Read the model definition and answer for the solid it produces. Units are mm, in the model's axes. A direction names the side the tool comes from. Coordinates: 2 decimals unless noted, no trailing zeros. Write each loop counter-clockwise with the first axis right and the second up, starting at its lowest first coordinate (ties: lowest second). Pieces come first, ordered by that corner, then holes. Notation, with made-up numbers: (-34.5, 71) -> (9.5, 71) arc R29 cw to (9.5, 110) -> close; hole circle Ø9 at (68, 62). An arc over 180 degrees is marked (long way). Return JSON: item names as keys, results as strings.
from build123d import *

# Parameters (mm, degrees)
F0_W     = 38.1
F0_H     = 25.4
F1_DEPTH = 12.7
F2_W     = 25.409764
F2_H     = 17.182311
F3_DEPTH = 25.401
F5_DEPTH = 38.101


with BuildPart() as f1:
    # F0 (on Front) → F1 (new body, symmetric)
    with BuildSketch(Plane.XZ):
        with Locations((19.05, 12.7)):
            Rectangle(F0_W, F0_H)
    extrude(amount=F1_DEPTH, both=True)

    # F2 (on face) → F3 (cut, through all)
    with BuildSketch(Plane.XZ.offset(12.7)):
        with Locations((25.395118, 16.808844)):
            Rectangle(F2_W, F2_H)
    extrude(amount=-F3_DEPTH, mode=Mode.SUBTRACT)

    # F4 (on face) → F5 (cut, through all)
    with BuildSketch(Plane(origin=(0, 0, 0), x_dir=(0, -1, 0), z_dir=(-1, 0, 0))):
        with BuildLine():
            ThreePointArc((-12.7, 12.223971), (0, 24.601783), (12.7, 12.223971))
            Line((12.7, 12.223971), (12.7, 25.4))
            Line((12.7, 25.4), (-12.7, 25.4))
            Line((-12.7, 25.4), (-12.7, 12.223971))
        make_face()
    extrude(amount=-F5_DEPTH, mode=Mode.SUBTRACT)


solid = f1.part
1. A tool of negligible diameter and unlimited length cuts with its end or side. For faces 1 (the face through (19, -12.7, 5)), 2 (the face through (25, 0, 8.218)), from which of +Z, -Z, +X, -X, +Y, -Y can it reach the whole face along a straight path? Write none if from no direction.
Taken from the geometry:
{"face 1": "+Z, -Z, +X, -X, -Y", "face 2": "+Z, +X, +Y, -Y"}
2. A flat-ended cylindrical pin translates along its axis: pin 1 Ø8 at (y, z) = (-4.5, 17) entering from +X. Find the tip coordinate at first contact, or state that the pin passes through.
Taken from the geometry:
{"pin 1": "stops at x = 12.69"}
3. The part is cut by section C-C (z = 15.5). Determine the outline of the cut face in (x, y), then the cut area to 3 significant figures.
Taken from the geometry:
{"outline": "(0, -12.18) -> (12.69, -12.18) -> (12.69, 12.18) -> (0, 12.18) -> close", "area": "309 mm2"}
4. Consider L1, parallel to Z at x = 28.5, y = 3.5; L2, parallel to X at y = 0.75, z = 14.5; L3, parallel to Y at x = 8.5, z = 12.5. Determine where each line is inside the solid, lowest interval first.
Taken from the geometry:
{"L1": "z = 0 to 8.22", "L2": "x = 0 to 12.69", "L3": "y = -12.69 to 12.69"}
5. The part is cut by section A-A (y = 0). Determine the outline of the cut face in (x, z), then the cut area to 3 significant figures.
Taken from the geometry:
{"outline": "(0, 0) -> (38.1, 0) -> (38.1, 8.22) -> (12.69, 8.22) -> (12.69, 24.6) -> (0, 24.6) -> close", "area": "521 mm2"}
6. The part is cut by section D-D (y = -6.75). Determine the outline of the cut face in (x, z), then the cut area to 3 significant figures.
Taken from the geometry:
{"outline": "(0, 0) -> (38.1, 0) -> (38.1, 8.22) -> (12.69, 8.22) -> (12.69, 22.66) -> (0, 22.66) -> close", "area": "496 mm2"}
